Source: CAD feature listing. Evaluate the final solid. Frame: model axes, mm. A direction names the side the tool comes from. Round coordinates to 2 decimals unless told otherwise and drop trailing zeros. Write each loop counter-clockwise with the first axis right and the second up, starting at its lowest first coordinate (ties: lowest second). Pieces come first, ordered by that corner, then holes.
from build123d import *

# Parameters (mm, degrees)
SKETCH_R   = 1.1
SKETCH_R_2 = 3.75
PAD_DEPTH  = 5


with BuildPart() as part:
    # Sketch → Pad (new body)
    with BuildSketch(Plane.XY):
        with BuildLine():
            Line((-152.2, 62.598999), (-152.2, 44.092341))
            Line((-127.2, 44.092341), (-152.2, 44.092341))
            Line((-127.2, 30.892341), (-127.2, 44.092341))
            Line((-152.2, 30.892341), (-127.2, 30.892341))
            Line((-152.2, 30.892341), (-152.2, 12.001349))
            ThreePointArc((-152.2, 12.001349), (-148.833331, 3.256809), (-140.206767, -0.401585))
            Line((-140.206767, -0.401585), (-108.826601, -0.401585))
            Line((-108.826601, 4), (-108.826601, -0.401585))
            Line((-98.826601, 4), (-108.826601, 4))
            Line((-98.826601, 0), (-98.826601, 4))
            Line((-98.826601, 0), (-72.233324, 0))
            Line((-72.233324, 4), (-72.233324, 0))
            Line((-62.233324, 4), (-72.233324, 4))
            Line((-62.233324, 0), (-62.233324, 4))
            Line((-62.233324, 0), (-35.826601, 0))
            Line((-35.826601, 4), (-35.826601, 0))
            Line((-25.826601, 4), (-35.826601, 4))
            Line((-25.826601, 0), (-25.826601, 4))
            Line((-25.826601, 0), (5.867454, -0.117862))
            ThreePointArc((5.867454, -0.117862), (14.389845, 3.441069), (17.86, 11.999991))
            Line((17.86, 25.499993), (17.86, 11.999991))
            Line((17.86, 25.499993), (-12.05, 25.499993))
            ThreePointArc((-12.050007, 49.499989), (-24.049998, 37.499988), (-12.05, 25.499993))
            Line((17.8, 49.500007), (-12.050007, 49.499989))
            Line((17.8, 49.500007), (17.8, 62.599011))
            ThreePointArc((17.8, 62.599011), (14.433945, 71.344583), (5.806821, 75.003556))
            Line((5.806821, 75.003556), (-25.826601, 75.003556))
            Line((-25.826601, 71), (-25.826601, 75.003556))
            Line((-35.826601, 71), (-25.826601, 71))
            Line((-35.826601, 75), (-35.826601, 71))
            Line((-35.826601, 75), (-62.326601, 75))
            Line((-62.326601, 71), (-62.326601, 75))
            Line((-72.326601, 71), (-62.326601, 71))
            Line((-72.326601, 75), (-72.326601, 71))
            Line((-72.326601, 75), (-98.82, 75))
            Line((-98.82, 71.087749), (-98.82, 75))
            Line((-108.82, 71.087749), (-98.82, 71.087749))
            Line((-108.82, 75.087749), (-108.82, 71.087749))
            Line((-108.82, 75.087749), (-140.32794, 74.598317))
            ThreePointArc((-140.32794, 74.598317), (-148.730395, 71.038925), (-152.2, 62.598999))
        make_face()
        with Locations((5.962192, 55.25)):
            Circle(SKETCH_R, mode=Mode.SUBTRACT)
        with Locations((-65.037808, 55.25)):
            Circle(SKETCH_R, mode=Mode.SUBTRACT)
        with Locations((-65.037808, 19.75)):
            Circle(SKETCH_R, mode=Mode.SUBTRACT)
        with Locations((5.962192, 19.75)):
            Circle(SKETCH_R, mode=Mode.SUBTRACT)
        with Locations((-140.2, 62.598999)):
            Circle(SKETCH_R, mode=Mode.SUBTRACT)
        with Locations((-140.206767, 11.598415)):
            Circle(SKETCH_R, mode=Mode.SUBTRACT)
        with Locations((5.860579, 11.882136)):
            Circle(SKETCH_R, mode=Mode.SUBTRACT)
        with Locations((5.806821, 63.003556)):
            Circle(SKETCH_R, mode=Mode.SUBTRACT)
        with Locations((-115.261171, 37.5)):
            Circle(SKETCH_R_2, mode=Mode.SUBTRACT)
        with Locations((-115.261171, 56.25)):
            Circle(SKETCH_R_2, mode=Mode.SUBTRACT)
        with Locations((-115.261171, 18.75)):
            Circle(SKETCH_R_2, mode=Mode.SUBTRACT)
    extrude(amount=PAD_DEPTH)


solid = part.part
1) Section query B-B on z = 2.25. State how many separate pieces and enclosed holes the cut face has, then the cut area to 3 significant figures.
Taken from the geometry:
separate pieces: 1
enclosed holes: 11
area: 11,000 mm2
2) Pull-direction query (Y, two-part tool) for faces 3 (the face through (-25.827, 73, 2)), 4 (the face through (-10, 75.004, 2)), 5 (the face through (-118.24, 16.47, 2.46)); classes: released by +Y, released by -Y, zero draft, split by the parting line, or undercut.
Taken from the geometry:
face 3: zero draft
face 4: released by +Y
face 5: undercut
3) Contact query for flat-ended pins moving along their axis: P1, Ø1.5, axis at x = -60, z = 4.5, coming from the +Y side; P2, Ø2, axis at x = -140.2, y = 62.599, coming from the +Z side; P3, Ø3, axis at y = 72, z = 2, coming from the -X side; P4, Ø2, axis at y = 1, z = 3, coming from the +X side. Output: stop coordinate, or through.
Taken from the geometry:
P1: stops at y = 75
P2: passes through
P3: stops at x = -149.23
P4: stops at x = 12.67
4) Material intervals for line 1 (X direction, y = 11, z = 1.65); line 2 (Y direction, x = 3.5, z = 3.55); line 3 (X direction, y = 63, z = 3.05), sorted ascending.
Taken from the geometry:
line 1: x = -152.19 to -141.13, -139.28 to 5.2, 6.52 to 17.83
line 2: y = -0.11 to 25.5, 49.5 to 75
line 3: x = -152.19 to -141.22, -139.18 to 4.71, 6.91 to 17.81
5) Reachability of faces 1 (the face through (-62.327, 73, 2)), 2 (the face through (-108.827, 2, 2)) from +Z, -Z, +X, -X, +Y, -Y: full face, straight path, thin tool, end or side. Return the list, or none.
Taken from the geometry:
face 1: +Z, -Z, +Y
face 2: +Z, -Z, -Y
6) Section query A-A on y = 37.5. Return the cut outline in (x, z).
Taken from the geometry:
outline: (-127.2, 0) - (-119.01, 0) - (-119.01, 5) - (-127.2, 5) - close; (-111.51, 0) - (-24.05, 0) - (-24.05, 5) - (-111.51, 5) - close
7) Section query D-D on x = -101. Return the cut outline in (y, z), then the cut area to 3 significant figures.
Taken from the geometry:
outline: (4, 0) - (71.09, 0) - (71.09, 5) - (4, 5) - close
area: 335 mm2
8) Section query C-C on x = -33.5. Return the cut outline in (y, z).
Taken from the geometry:
outline: (4, 0) - (71, 0) - (71, 5) - (4, 5) - close
